Read the model definition and answer for the solid it produces. Units are mm, in the model's axes. Give positions to 0.01 mm unless a question says otherwise; leave off trailing zeros. Order: outer loops, then holes, each group sorted by start corner. A loop starts at its lowest first (then second) coordinate and runs counter-clockwise, first axis right, second up.
Item 1: Given pin 1 Ø3 at (x, y) = (72.5, 14) entering from +Z; pin 2 Ø4 at (x, y) = (36.5, 2.5) entering from -Z, each flat-ended and moving along its own axis, determine where each tip first touches the part or whether it passes through.
Item 2: Find the intervals of material crossed by line 1 along Z through (x, y) = (49, 10.75); line 2 along Z through (x, y) = (69, 17); line 3 along X through (y, z) = (7.5, -612), in increasing order.
Item 3: A cutting plane is placed at B-B (x = 88). Write down the section's boundary in (y, z).
Item 4: The mould has two halves that part along X. Classify faces 1 (the face through (37.993, 9.126, -286.753)), 2 (the face through (0, 9, -296)), 3 (the face through (51, 0, -294)): +X half, -X half, draft (parallel to the pull), parting line (faces both ways), or undercut.
Item 5: A cutting plane is placed at A-A (y = 6). State how many separate pieces and enclosed holes the cut face has, plus the area to 3 significant figures.
Item 6: A cutting plane is placed at C-C (z = 44.5). Write down the section's boundary in (x, y), plus the area to 3 significant figures.
Autodesk Inventor part; units mm, degrees
ref_plane "YZ Plane" through (0, 0, 0) normal (1, 0, 0) x (0, 1, 0)
ref_plane "XZ Plane" through (0, 0, 0) normal (0, 1, 0) x (-1, 0, 0)
ref_plane "XY Plane" through (0, 0, 0) normal (0, 0, 1) x (1, 0, 0)
sketch "Sketch1" plane through (0, 0, 0) normal (0, 1, 0) x (-1, 0, 0)
  line L0 (0, 0) -> (0, -600)
  line L1 (0, 0) -> (-100, 0)
  line L2 (-100, 0) -> (-100, 100)
  line L3 (-100, 100) -> (0, 0)
  line L4 (0, -600) -> (-100, -600)
  line L5 (-100, -600) -> (-100, -700)
  line L6 (-100, -700) -> (0, -600)
  line L7 (-100, -600) -> (-100, 0)
  dimension "d0" = 600
  dimension "d1" = 100
  dimension "d2" = 100
  dimension "d3" = 100
  dimension "d4" = 100
extrude "Extrusion1" add sketch "Sketch1" along normal blind 18
sketch "Sketch3" plane through (0, 18, 0) normal (0, 1, 0) x (1, 0, 0)
  circle A0 centre (38.9698, 279.3172) radius 7.5
  line L0 (100, 700) -> (0, 600)
  line L1 (0, 0) -> (100, -100)
  line L2 (0, 0) -> (100, -100)
  line L3 (100, -100) -> (100, 700)
  line L4 (100, 700) -> (0, 600)
  line L5 (0, 600) -> (0, 0)
extrude "Extrusion2" cut sketch "Sketch3" against normal blind 20 contours A0
sketch "Sketch4" plane through (0, 0, 0) normal (0, -1, 0) x (1, 0, 0)
  circle A0 centre (38.9698, -279.3172) radius 7.5
  line L0 (100, 100) -> (100, -700)
  line L1 (17.2005, -615) -> (17.2005, 25)
  line L2 (22.2005, -326.9779) -> (47.2005, -326.9779)
  line L3 (47.2005, -326.9779) -> (47.2005, -391.9779)
  line L4 (47.2005, -391.9779) -> (22.2005, -391.9779)
  line L5 (0, -600) -> (0, 0)
  line L6 (100, -700) -> (0, -600)
  line L7 (0, 0) -> (100, 100)
  circle A1 centre (38.9698, -279.3539) radius 7.5
  circle A2 centre (38.9698, -279.3539) radius 4.625
  circle A3 centre (38.9698, -279.3539) radius 5.75
  circle A4 centre (38.7754, -333.8918) radius 1
  circle A5 centre (34.7754, -333.8918) radius 1
  circle A6 centre (30.7754, -333.8918) radius 1
  circle A7 centre (38.7754, -337.8918) radius 1
  circle A8 centre (34.7754, -337.8918) radius 1
  circle A9 centre (30.7754, -337.8918) radius 1
  circle A10 centre (38.7754, -341.8918) radius 1
  circle A11 centre (34.7754, -341.8918) radius 1
  circle A12 centre (30.7754, -341.8918) radius 1
  circle A13 centre (38.7005, -377.1197) radius 1
  circle A14 centre (34.7005, -377.1197) radius 1
  circle A15 centre (30.7005, -377.1197) radius 1
  circle A16 centre (38.7005, -381.1197) radius 1
  circle A17 centre (34.7005, -381.1197) radius 1
  circle A18 centre (30.7005, -381.1197) radius 1
  circle A19 centre (38.7005, -385.1197) radius 1
  circle A20 centre (34.7005, -385.1197) radius 1
  circle A21 centre (30.7005, -385.1197) radius 1
  dimension "d9" = 2
  dimension "d12" = 4
  dimension "d15" = 4
  dimension "d18" = 2
  dimension "d19" = 4
  dimension "d20" = 4
extrude "Extrusion3" cut sketch "Sketch4" against normal blind 20 contours A4 | A5 | A6 | A7 | A8 | A9 | A10 | A11 | A12 | A13 | A14 | A15 | A16 | A17 | A18 | A19 | A20 | A21
properties part number "Fata_4"
Response values:
1. pin 1: stops at z = 74
1. pin 2: stops at z = -638.5
2. line 1: z = -649 to 49
2. line 2: z = -669 to 69
2. line 3: x = 12 to 100
3. outline: (0, -688) - (18, -688) - (18, 88) - (0, 88) - close
4. face 1: undercut
4. face 2: -X half
4. face 3: draft
5. separate pieces: 1
5. enclosed holes: 19
5. area: 69,800 mm2
6. outline: (44.5, 0) - (100, 0) - (100, 18) - (44.5, 18) - close
6. area: 999 mm2
